Could you check a few things on this drawing? It's one solid part, dimensions in mm from its lowest x, y, z. A direction names the side the tool comes from. Coordinates: 2 decimals unless noted, no trailing zeros. Order: outer loops, then holes, each group sorted by start corner. A loop starts at its lowest first (then second) coordinate and runs counter-clockwise, first axis right, second up. Notation, with made-up numbers: (-12.5, 3.25) - (0.5, 3.25) arc R14 ccw to (0.5, 10.25) - close; hole circle Ø1 at (41, 78.25). An arc over 180 degrees is marked (long way). Answer in a Markdown table with one row per item. Add a question column.
Item 1: I want a section at A-A (x = 118). Please give me the cut outline in (y, z).
Item 2: If I drill on line 1 along Z through (x, y) = (101.5, 27.5); line 2 along X through (y, z) = (11.5, 30), over which ranges is the centre line in solid material (lowest first)? Write a range as from..to.
Item 3: Will these pins go through, and if not, where does the flat tip stop? pin 1 Ø2 at (y, z) = (10, 38.5) entering from +X; pin 2 Ø8 at (x, y) = (87.5, 28) entering from -Z; pin 3 Ø10 at (x, z) = (15, 41.5) entering from +Y.
Item 4: I want a section at B-B (y = 7). Please give me the cut outline in (x, z).
Item 5: On a 3-axis mill with a long thin cutter (end or side, diameter ignored), from which of +Z, -Z, +X, -X, +Y, -Y can I reach the whole of each face in a straight line? I mean the marked faces 1 and 2. Say none if no direction works.
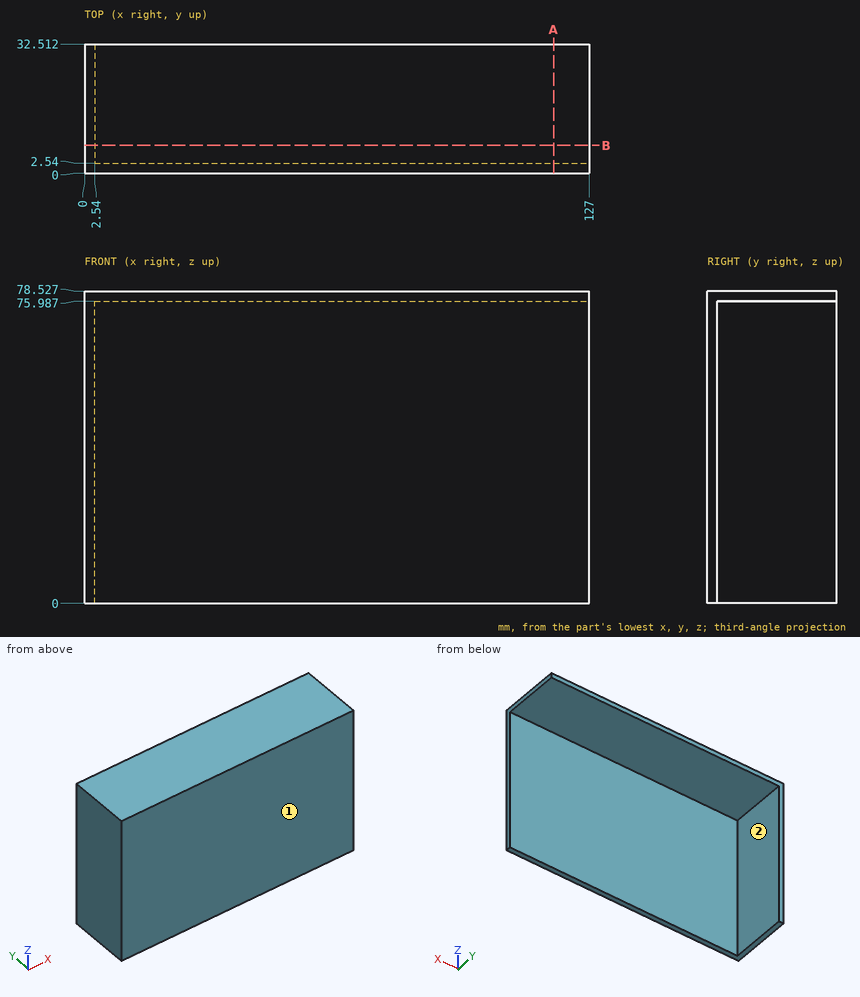
Values follow:
| question | item | result |
|---|---|---|
| 1 | outline | (0, 0) - (2.54, 0) - (2.54, 75.99) - (32.51, 75.99) - (32.51, 78.53) - (0, 78.53) - close |
| 2 | line 1 | z = 75.99..78.53 |
| 2 | line 2 | x = 0..2.54 |
| 3 | pin 1 | stops at x = 2.54 |
| 3 | pin 2 | stops at z = 75.99 |
| 3 | pin 3 | stops at y = 2.54 |
| 4 | outline | (0, 0) - (2.54, 0) - (2.54, 75.99) - (127, 75.99) - (127, 78.53) - (0, 78.53) - close |
| 5 | face 1 | +Z, -Z, +X, -X, -Y |
| 5 | face 2 | -Z, +X, +Y |
